Verification items for the finished model (mm, model axes). Face numbers are marked on the shaded views. A direction names the side the tool comes from. Round coordinates to 2 decimals unless told otherwise and drop trailing zeros. Write each loop counter-clockwise with the first axis right and the second up, starting at its lowest first coordinate (ties: lowest second). Pieces come first, ordered by that corner, then holes. Notation, with made-up numbers: M -9.5,-11 L 17.5,-11 A20 cw 17.5,-4 Z; hole C 85,38.25 d7. An arc over 180 degrees is marked long. Answer in a Markdown table with one row per item. Add a question column.
1. Sectioned sample at D-D on z = 33.5. Record the cut outline in (x, y).
2. Draft check along Y on the marked faces 4 and 5. Enter one of: pulls with the +Y half, pulls with the -Y half, needs draft (parallel to the pull), parting line crosses it, or undercut.
3. Sectioned sample at A-A on y = 15.5. Record the cut outline in (x, z), plus the area to 3 significant figures.
4. Material ranges on probe 1 along Y at (x, z) = (11.4, 8.5); probe 2 along Y at (x, z) = (-4, 20); probe 3 along Z at (x, y) = (-9.25, -5.5), recorded low to high.
5. Sectioned sample at B-B on y = 0. Record the cut outline in (x, z), plus the area to 3 significant figures.
6. Go/stop test with flat-tipped pins: pin 1 Ø1.5 at (x, z) = (-9.5, 0) entering from +Y; pin 2 Ø6 at (x, z) = (-7.5, 14) entering from -Y; pin 3 Ø5.5 at (y, z) = (14, 9.5) entering from -X; pin 4 Ø0.6 at (x, y) = (9, 1.5) entering from +Z. Record where each tip stops, or that it passes through.
7. Sectioned sample at C-C on z = 15. Record the cut outline in (x, y), plus the area to 3 significant figures.
8. Set-up check for the marked faces 1, 2 and 3: record each of +Z, -Z, +X, -X, +Y, -Y from which the full face is reachable in a straight line by a thin tool's end or side.
```python
from build123d import *

# Parameters (mm, degrees)
EXTRUDE_1_DEPTH      = 42
EXTRUDE_1_DEPTH_BACK = 10
SKETCH_1_W           = 24
SKETCH_1_H           = 24
SKETCH_3_R           = 10.5
CUT_EXTRUDE_1_DEPTH  = 20
SKETCH_4_W           = 17
SKETCH_4_H           = 17
CUT_EXTRUDE_2_DEPTH  = 29
SKETCH_5_W           = 17
SKETCH_5_H           = 17
CUT_EXTRUDE_5_DEPTH  = 50.839743178
SKETCH_6_W           = 7
SKETCH_6_H           = 7
SKETCH_6_R           = 1.5
EXTRUDE_2_DEPTH      = 2


with BuildPart() as part:
    # Эскиз1 → Бобышка-Вытянуть1 (new, two sides: drawn at the far end of the back side and taken through both)
    with BuildSketch(Plane.XY.offset(-EXTRUDE_1_DEPTH_BACK)):
        Rectangle(SKETCH_1_W, SKETCH_1_H)
    extrude(amount=EXTRUDE_1_DEPTH + EXTRUDE_1_DEPTH_BACK)

    # Эскиз3 → Вырез-Вытянуть1 (cut)
    with BuildSketch(Plane.XY.offset(42)):
        Circle(SKETCH_3_R)
    extrude(amount=-CUT_EXTRUDE_1_DEPTH, mode=Mode.SUBTRACT)

    # Эскиз4 → Вырез-Вытянуть2 (cut)
    with BuildSketch(Plane.XY.offset(22)):
        Rectangle(SKETCH_4_W, SKETCH_4_H)
    extrude(amount=-CUT_EXTRUDE_2_DEPTH, mode=Mode.SUBTRACT)

    # Эскиз5 → Вырез-Вытянуть5 (cut, through all)
    with BuildSketch(Plane(origin=(12, 0, 0), x_dir=(0, 0, -1), z_dir=(1, 0, 0))):
        with Locations((-8.5, 0)):
            Rectangle(SKETCH_5_W, SKETCH_5_H)
    extrude(amount=-CUT_EXTRUDE_5_DEPTH, mode=Mode.SUBTRACT)

    # Эскиз6 → Бобышка-Вытянуть2 (add)
    # profile 1 of 2: a face of its own
    with BuildSketch(Plane(origin=(12, 0, 0), x_dir=(0, 0, -1), z_dir=(1, 0, 0))):
        with Locations((-8.5, 15.5)):
            Rectangle(SKETCH_6_W, SKETCH_6_H)
        with Locations((-8.5, 15.5)):
            Circle(SKETCH_6_R, mode=Mode.SUBTRACT)
    # profile 2 of 2: a face of its own
    with BuildSketch(Plane(origin=(12, 0, 0), x_dir=(0, 0, -1), z_dir=(1, 0, 0))):
        with Locations((-8.5, -15.5)):
            Rectangle(SKETCH_6_W, SKETCH_6_H)
        with Locations((-8.5, -15.5)):
            Circle(SKETCH_6_R, mode=Mode.SUBTRACT)
    extrude(amount=-EXTRUDE_2_DEPTH)


solid = part.part
```
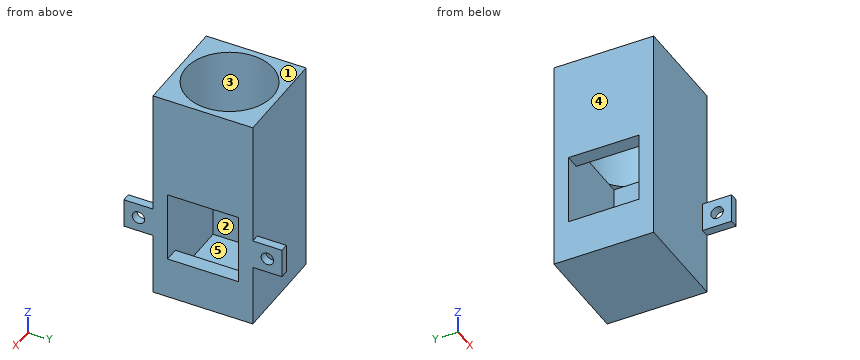
Geometry check:
| question | item | result |
|---|---|---|
| 1 | outline | M -12,-12 L 12,-12 L 12,12 L -12,12 Z; hole C 0,0 d21 |
| 2 | face 4 | needs draft |
| 2 | face 5 | undercut |
| 3 | outline | M 10,5 L 12,5 L 12,7 L 10,7 Z; M 10,10 L 12,10 L 12,12 L 10,12 Z |
| 3 | area | 8.00 mm2 |
| 4 | probe 1 | y = -19 to -17, -14 to -8.5, 8.5 to 14, 17 to 19 |
| 4 | probe 2 | y = -12 to -8.5, 8.5 to 12 |
| 4 | probe 3 | z = -10 to 0, 17 to 42 |
| 5 | outline | M -12,-10 L 12,-10 L 12,0 L 8.5,0 L 8.5,-7 L -8.5,-7 L -8.5,0 L -12,0 Z; M -12,17 L -8.5,17 L -8.5,22 L -10.5,22 L -10.5,42 L -12,42 Z; M 8.5,17 L 12,17 L 12,42 L 10.5,42 L 10.5,22 L 8.5,22 Z |
| 5 | area | 216 mm2 |
| 6 | pin 1 | stops at y = 12 |
| 6 | pin 2 | stops at y = -12 |
| 6 | pin 3 | stops at x = -12 |
| 6 | pin 4 | stops at z = 22 |
| 7 | outline | M -12,-12 L 12,-12 L 12,-8.5 L -12,-8.5 Z; M -12,8.5 L 12,8.5 L 12,12 L -12,12 Z |
| 7 | area | 168 mm2 |
| 8 | face 1 | +Z, +X, -X, +Y, -Y |
| 8 | face 2 | none |
| 8 | face 3 | +Z |
